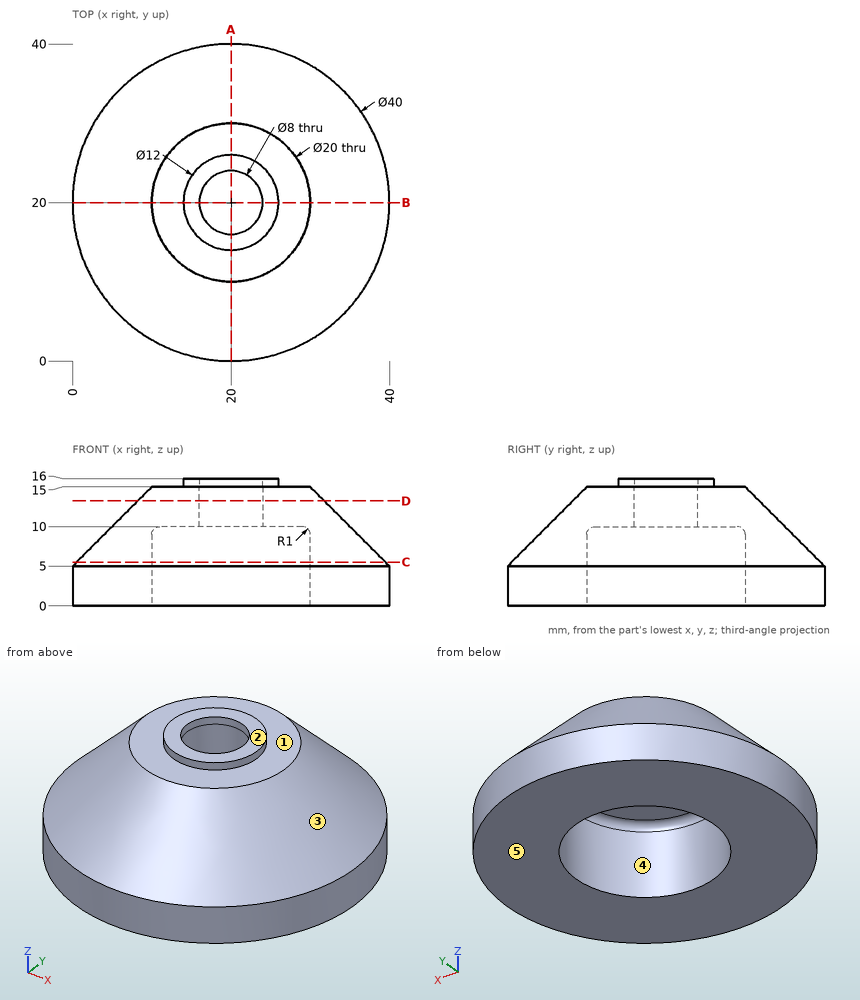
Study the drawing (mm; zero at the part's minimum x, y, z) and answer. A direction names the side the tool comes from. Round coordinates to 2 decimals unless told otherwise and drop trailing zeros. Write each loop counter-clockwise with the first axis right and the second up, starting at its lowest first coordinate (ties: lowest second). Pieces come first, ordered by that corner, then holes. Notation, with made-up numbers: (40.5, 6) -> (56.5, 6) arc R22 cw to (56.5, 38) -> close; hole circle Ø8 at (-8.5, 34). An arc over 180 degrees is marked (long way). Answer as CSV lines item,"result". Start each with the question number.
(1) The part is cut by section A-A, the plane x = 20. Give the vertices of the cut face in (y, z), then the cut area to 3 significant figures.
(2) The part is cut by section D-D, the plane z = 13.25. Give the vertices of the cut face in (x, y), then the cut area to 3 significant figures.
(3) The part is cut by section C-C, the plane z = 5.5. Give the vertices of the cut face in (x, y), then the cut area to 3 significant figures.
(4) A tool of negligible diameter and unlimited length cuts with its end or side. For the marked faces 1 and 2, from which of +Z, -Z, +X, -X, +Y, -Y can it reach the whole face along a straight path? Write none if from no direction.
(5) Each of these flat-tipped pins is pushed along its axis until it touches: pin 1 (6.5 mm diameter, centred on x = 20, y = 20, fed in from -Z); pin 2 (1.5 mm diameter, centred on x = 23, y = 22.5, fed in from -Z); pin 3 (1 mm diameter, centred on x = 26, z = 9.5, fed in from +Y); pin 4 (2 mm diameter, centred on y = 7, z = 9.5, fed in from +X). Where does it stop, or does it pass through?
(6) The mould has two halves that part along Y. Classify the marked faces 3, 4 and 5: +Y half, -Y half, draft (parallel to the pull), parting line (faces both ways), or undercut.
(7) Find the intervals of material crossed by probe 1 along Y at (x, z) = (20, 15.55); probe 2 along Y at (x, z) = (20, 11.6); probe 3 along Z at (x, y) = (23.5, 13), in increasing order.
Output values:
1,outline,"(0, 0) -> (10, 0) -> (10, 9) arc R1 cw to (11, 10) -> (16, 10) -> (16, 16) -> (14, 16) -> (14, 15) -> (10, 15) -> (0, 5) -> close; (24, 10) -> (29, 10) arc R1 cw to (30, 9) -> (30, 0) -> (40, 0) -> (40, 5) -> (30, 15) -> (26, 15) -> (26, 16) -> (24, 16) -> close"
1,area,"264 mm²"
2,outline,"circle Ø23.5 at (20, 20); hole circle Ø8 at (20, 20)"
2,area,"383 mm²"
3,outline,"circle Ø39 at (20, 20); hole circle Ø20 at (20, 20)"
3,area,"880 mm²"
4,face 1,"+Z"
4,face 2,"+Z, +X, -X, +Y, -Y"
5,pin 1,"passes through"
5,pin 2,"stops at z = 10"
5,pin 3,"stops at y = 34.87"
5,pin 4,"stops at x = 30.58"
6,face 3,"parting line"
6,face 4,"undercut"
6,face 5,"draft"
7,probe 1,"y = 14 to 16, 24 to 26"
7,probe 2,"y = 6.6 to 16, 24 to 33.4"
7,probe 3,"z = 10 to 15"
